```python
from build123d import *

# Parameters (mm, degrees)
SKETCH1_R               = 1.5
BOSS_EXTRUDE1_DEPTH     = 206
CUT_EXTRUDE1_DEPTH      = 10
CUT_EXTRUDE1_DEPTH_BACK = 10
SKETCH2_R               = 1.5
CUT_EXTRUDE2_DEPTH      = 10
CUT_EXTRUDE2_DEPTH_BACK = 10
SKETCH4_R               = 1.5


with BuildPart() as part:
    # Sketch1 → Boss-Extrude1 (new body)
    with BuildSketch(Plane(origin=(0, 0, 0), x_dir=(1, 0, 0), z_dir=(0, 1, 0))):
        with BuildLine():
            Line((-10, 4.65), (-9.8, 4.65))
            Line((-9.8, 4.65), (-9.8, 4.4))
            ThreePointArc((-9.8, 4.4), (-9.741421356, 4.258578644), (-9.6, 4.2))
            Line((-9.6, 4.2), (-8.4, 4.2))
            ThreePointArc((-8.4, 4.2), (-8.258578644, 4.258578644), (-8.2, 4.4))
            Line((-8.2, 4.4), (-8.2, 5.45))
            ThreePointArc((-8.2, 5.45), (-8.141421356, 5.591421356), (-8, 5.65))
            Line((-8, 5.65), (-6.832842712, 5.65))
            ThreePointArc((-6.832842712, 5.65), (-6.756306026, 5.634775907), (-6.691421356, 5.591421356))
            Line((-6.691421356, 5.591421356), (-4.058578644, 2.958578644))
            ThreePointArc((-4.058578644, 2.958578644), (-4.015224093, 2.893693974), (-4, 2.817157288))
            Line((-4, 2.817157288), (-4, -2.817157288))
            ThreePointArc((-4, -2.817157288), (-4.015224093, -2.893693974), (-4.058578644, -2.958578644))
            Line((-4.058578644, -2.958578644), (-6.691421356, -5.591421356))
            ThreePointArc((-6.691421356, -5.591421356), (-6.756306026, -5.634775907), (-6.832842712, -5.65))
            Line((-6.832842712, -5.65), (-8, -5.65))
            ThreePointArc((-8, -5.65), (-8.141421356, -5.591421356), (-8.2, -5.45))
            Line((-8.2, -5.45), (-8.2, -4.4))
            ThreePointArc((-8.2, -4.4), (-8.258578644, -4.258578644), (-8.4, -4.2))
            Line((-8.4, -4.2), (-9.6, -4.2))
            ThreePointArc((-9.6, -4.2), (-9.741421356, -4.258578644), (-9.8, -4.4))
            Line((-9.8, -4.4), (-9.8, -4.65))
            Line((-9.8, -4.65), (-10, -4.65))
            Line((-10, -4.65), (-10, -9.8))
            ThreePointArc((-10, -9.8), (-9.941421356, -9.941421356), (-9.8, -10))
            Line((-9.8, -10), (-4.65, -10))
            Line((-4.65, -10), (-4.65, -9.8))
            Line((-4.65, -9.8), (-4.4, -9.8))
            ThreePointArc((-4.4, -9.8), (-4.258578644, -9.741421356), (-4.2, -9.6))
            Line((-4.2, -9.6), (-4.2, -8.4))
            ThreePointArc((-4.2, -8.4), (-4.258578644, -8.258578644), (-4.4, -8.2))
            Line((-4.4, -8.2), (-5.45, -8.2))
            ThreePointArc((-5.45, -8.2), (-5.591421356, -8.141421356), (-5.65, -8))
            Line((-5.65, -8), (-5.65, -6.832842712))
            ThreePointArc((-5.65, -6.832842712), (-5.634775907, -6.756306026), (-5.591421356, -6.691421356))
            Line((-5.591421356, -6.691421356), (-2.958578644, -4.058578644))
            ThreePointArc((-2.958578644, -4.058578644), (-2.893693974, -4.015224093), (-2.817157288, -4))
            Line((-2.817157288, -4), (2.817157288, -4))
            ThreePointArc((2.817157288, -4), (2.893693974, -4.015224093), (2.958578644, -4.058578644))
            Line((2.958578644, -4.058578644), (5.591421356, -6.691421356))
            ThreePointArc((5.591421356, -6.691421356), (5.634775907, -6.756306026), (5.65, -6.832842712))
            Line((5.65, -6.832842712), (5.65, -8))
            ThreePointArc((5.65, -8), (5.591421356, -8.141421356), (5.45, -8.2))
            Line((5.45, -8.2), (4.4, -8.2))
            ThreePointArc((4.4, -8.2), (4.258578644, -8.258578644), (4.2, -8.4))
            Line((4.2, -8.4), (4.2, -9.6))
            ThreePointArc((4.2, -9.6), (4.258578644, -9.741421356), (4.4, -9.8))
            Line((4.4, -9.8), (4.65, -9.8))
            Line((4.65, -9.8), (4.65, -10))
            Line((4.65, -10), (9.8, -10))
            ThreePointArc((9.8, -10), (9.941421356, -9.941421356), (10, -9.8))
            Line((10, -9.8), (10, -4.65))
            Line((10, -4.65), (9.8, -4.65))
            Line((9.8, -4.65), (9.8, -4.4))
            ThreePointArc((9.8, -4.4), (9.741421356, -4.258578644), (9.6, -4.2))
            Line((9.6, -4.2), (8.4, -4.2))
            ThreePointArc((8.4, -4.2), (8.258578644, -4.258578644), (8.2, -4.4))
            Line((8.2, -4.4), (8.2, -5.45))
            ThreePointArc((8.2, -5.45), (8.141421356, -5.591421356), (8, -5.65))
            Line((8, -5.65), (6.832842712, -5.65))
            ThreePointArc((6.832842712, -5.65), (6.756306026, -5.634775907), (6.691421356, -5.591421356))
            Line((6.691421356, -5.591421356), (4.058578644, -2.958578644))
            ThreePointArc((4.058578644, -2.958578644), (4.015224093, -2.893693974), (4, -2.817157288))
            Line((4, -2.817157288), (4, 2.817157288))
            ThreePointArc((4, 2.817157288), (4.015224093, 2.893693974), (4.058578644, 2.958578644))
            Line((4.058578644, 2.958578644), (6.691421356, 5.591421356))
            ThreePointArc((6.691421356, 5.591421356), (6.756306026, 5.634775907), (6.832842712, 5.65))
            Line((6.832842712, 5.65), (8, 5.65))
            ThreePointArc((8, 5.65), (8.141421356, 5.591421356), (8.2, 5.45))
            Line((8.2, 5.45), (8.2, 4.4))
            ThreePointArc((8.2, 4.4), (8.258578644, 4.258578644), (8.4, 4.2))
            Line((8.4, 4.2), (9.6, 4.2))
            ThreePointArc((9.6, 4.2), (9.741421356, 4.258578644), (9.8, 4.4))
            Line((9.8, 4.4), (9.8, 4.65))
            Line((9.8, 4.65), (10, 4.65))
            Line((10, 4.65), (10, 9.8))
            ThreePointArc((10, 9.8), (9.941421356, 9.941421356), (9.8, 10))
            Line((9.8, 10), (4.65, 10))
            Line((4.65, 10), (4.65, 9.8))
            Line((4.65, 9.8), (4.4, 9.8))
            ThreePointArc((4.4, 9.8), (4.258578644, 9.741421356), (4.2, 9.6))
            Line((4.2, 9.6), (4.2, 8.4))
            ThreePointArc((4.2, 8.4), (4.258578644, 8.258578644), (4.4, 8.2))
            Line((4.4, 8.2), (5.45, 8.2))
            ThreePointArc((5.45, 8.2), (5.591421356, 8.141421356), (5.65, 8))
            Line((5.65, 8), (5.65, 6.832842712))
            ThreePointArc((5.65, 6.832842712), (5.634775907, 6.756306026), (5.591421356, 6.691421356))
            Line((5.591421356, 6.691421356), (2.958578644, 4.058578644))
            ThreePointArc((2.958578644, 4.058578644), (2.893693974, 4.015224093), (2.817157288, 4))
            Line((2.817157288, 4), (-2.817157288, 4))
            ThreePointArc((-2.817157288, 4), (-2.893693974, 4.015224093), (-2.958578644, 4.058578644))
            Line((-2.958578644, 4.058578644), (-5.591421356, 6.691421356))
            ThreePointArc((-5.591421356, 6.691421356), (-5.634775907, 6.756306026), (-5.65, 6.832842712))
            Line((-5.65, 6.832842712), (-5.65, 8))
            ThreePointArc((-5.65, 8), (-5.591421356, 8.141421356), (-5.45, 8.2))
            Line((-5.45, 8.2), (-4.4, 8.2))
            ThreePointArc((-4.4, 8.2), (-4.258578644, 8.258578644), (-4.2, 8.4))
            Line((-4.2, 8.4), (-4.2, 9.6))
            ThreePointArc((-4.2, 9.6), (-4.258578644, 9.741421356), (-4.4, 9.8))
            Line((-4.4, 9.8), (-4.65, 9.8))
            Line((-4.65, 9.8), (-4.65, 10))
            Line((-4.65, 10), (-9.8, 10))
            ThreePointArc((-9.8, 10), (-9.941421356, 9.941421356), (-10, 9.8))
            Line((-10, 9.8), (-10, 4.65))
        make_face()
        with Locations(Location((0, 0, 0), (0, 0, 270))):
            Circle(SKETCH1_R, mode=Mode.SUBTRACT)
    extrude(amount=BOSS_EXTRUDE1_DEPTH)

    # Sketch2 → Cut-Extrude1 (cut, two sides: drawn at the far end of the back side and taken through both)
    with BuildSketch(Plane(origin=(4, 0, 0), x_dir=(0, 0, -1), z_dir=(1, 0, 0)).offset(-CUT_EXTRUDE1_DEPTH_BACK)):
        with Locations((0, 103)):
            Circle(SKETCH2_R)
    extrude(amount=CUT_EXTRUDE1_DEPTH + CUT_EXTRUDE1_DEPTH_BACK, mode=Mode.SUBTRACT)

    # Sketch4 → Cut-Extrude2 (cut, two sides: drawn at the far end of the back side and taken through both)
    with BuildSketch(Plane.XY.offset(4).offset(-CUT_EXTRUDE2_DEPTH_BACK)):
        with Locations(Location((0, 103, 0), (0, 0, 180))):
            Circle(SKETCH4_R)
    extrude(amount=CUT_EXTRUDE2_DEPTH + CUT_EXTRUDE2_DEPTH_BACK, mode=Mode.SUBTRACT)


solid = part.part
```
Part model, mm, in its own coordinate system. A direction names the side the tool comes from. Round coordinates to 2 decimals unless told otherwise and drop trailing zeros. Put each result on its own line as item: value. Start each with the question number.
1. Drop flat-ended pins along their axis: pin 1 (12 mm diameter, centred on x = 0.5, z = 7.5, fed in from +Y); pin 2 (1 mm diameter, centred on x = -3.5, y = 183.5, fed in from -Z); pin 3 (5 mm diameter, centred on x = 2, y = 35.5, fed in from +Z); pin 4 (1 mm diameter, centred on y = 145.5, z = -4, fed in from +X). Give the stop position or say it passes through.
2. Two-plate mould, pull along X, no slides. Class faces 1 (the face through (-1.2, 101.6, -4)), 2 (the face through (2, 206, 0)), 3 (the face through (4, 101.6, -1.2)): +X half, -X half, draft (parallel to the pull), parting line (faces both ways), or undercut.
3. Tool access for faces 4 (the face through (1.2, 101.6, 4)), 5 (the face through (-4, 101.6, 1.2)), 6 (the face through (-10, 102, -7)): list every direction of +Z, -Z, +X, -X, +Y, -Y with a clear straight run to the whole face (end or side of a thin tool).
4. Drill centre lines: probe 1 along X at (y, z) = (178.5, 0); probe 2 along Y at (x, z) = (-1.8, 0). Where is each one in solid material? Low to high. Write a range as [from, to].
Findings:
1. pin 1: y = 206
1. pin 2: z = -5.1
1. pin 3: z = 9.8
1. pin 4: x = 9.8
2. face 1: undercut
2. face 2: draft
2. face 3: +X half
3. face 4: +Z, +Y, -Y
3. face 5: -X, +Y, -Y
3. face 6: +Z, -Z, -X, +Y, -Y
4. probe 1: [-4, -1.5], [1.5, 4]
4. probe 2: [0, 101.5], [104.5, 206]
